from build123d import *

# Parameters (mm, degrees)
SKETCH2_W           = 208
SKETCH2_H           = 54
BOSS_EXTRUDE1_DEPTH = 10
SKETCH4_W           = 139
SKETCH4_H           = 54
CUT_EXTRUDE1_DEPTH  = 8
SKETCH3_W           = 40
SKETCH3_H           = 41
CUT_EXTRUDE2_DEPTH  = 8
SKETCH6_W           = 25
SKETCH6_H           = 54
BOSS_EXTRUDE2_DEPTH = 5
SKETCH7_W           = 20
SKETCH7_H           = 50
CUT_EXTRUDE3_DEPTH  = 1.5


with BuildPart() as part:
    # Sketch2 → Boss-Extrude1 (new body)
    with BuildSketch(Plane(origin=(0, 0, 0), x_dir=(1, 0, 0), z_dir=(0, 1, 0))):
        Rectangle(SKETCH2_W, SKETCH2_H)
    extrude(amount=BOSS_EXTRUDE1_DEPTH)

    # Sketch4 → Cut-Extrude1 (cut)
    with BuildSketch(Plane(origin=(0, 10, 0), x_dir=(1, 0, 0), z_dir=(0, 1, 0))):
        with Locations((-9.5, 0)):
            Rectangle(SKETCH4_W, SKETCH4_H)
    extrude(amount=-CUT_EXTRUDE1_DEPTH, mode=Mode.SUBTRACT)

    # Sketch3 → Cut-Extrude2 (cut)
    with BuildSketch(Plane(origin=(0, 10, 0), x_dir=(1, 0, 0), z_dir=(0, 1, 0))):
        with Locations((82, 2)):
            Rectangle(SKETCH3_W, SKETCH3_H)
    extrude(amount=-CUT_EXTRUDE2_DEPTH, mode=Mode.SUBTRACT)

    # Sketch6 → Boss-Extrude2 (add)
    with BuildSketch(Plane(origin=(0, 10, 0), x_dir=(1, 0, 0), z_dir=(0, 1, 0))):
        with Locations((-91.5, 0)):
            Rectangle(SKETCH6_W, SKETCH6_H)
    extrude(amount=BOSS_EXTRUDE2_DEPTH)

    # Sketch7 → Cut-Extrude3 (cut)
    with BuildSketch(Plane(origin=(0, 15, 0), x_dir=(1, 0, 0), z_dir=(0, 1, 0))):
        with Locations((-92, 0)):
            Rectangle(SKETCH7_W, SKETCH7_H)
    extrude(amount=-CUT_EXTRUDE3_DEPTH, mode=Mode.SUBTRACT)


solid = part.part
The listing builds one solid part. Answer for the finished solid, in the listing's coordinates (mm). A direction names the side the tool comes from. Give positions to 0.01 mm unless a question says otherwise; leave off trailing zeros. Loops run counter-clockwise (first coordinate to the right, second up) from the corner with the lowest first, then second, coordinate; pieces in that order, holes last.
Item 1: A tool of negligible diameter and unlimited length cuts with its end or side. For faces 1 (the flat face through (82, 10, 20)), 2 (the flat face through (82, 6, 18.5)), 3 (the flat face through (-79, 8, 0)), from which of +Z, -Z, +X, -X, +Y, -Y can it reach the whole face along a straight path? Write none if from no direction.
Derived:
face 1: +Z, -Z, +X, +Y
face 2: +Y
face 3: +Z, -Z, +Y
Item 2: Determine the mould class of faces 4 (the flat face through (82, 2, -2)), 5 (the flat face through (60, 6, 0)), 6 (the flat face through (0, 1, -27)) for opening direction Z: +Z half, -Z half, draft (parallel to the pull), parting line (faces both ways), or undercut.
Derived:
face 4: undercut
face 5: draft
face 6: -Z half
Item 3: Each of these flat-tipped pins is pushed along its axis until it touches: pin 1 Ø12 at (x, z) = (-83, -3) entering from +Y; pin 2 Ø10 at (x, z) = (-91, 6) entering from +Y; pin 3 Ø20 at (x, z) = (81.5, 5) entering from +Y; pin 4 Ø1.6 at (y, z) = (14, 3) entering from +X. Where does it stop, or does it pass through?
Derived:
pin 1: stops at y = 15
pin 2: stops at y = 13.5
pin 3: stops at y = 2
pin 4: stops at x = -79
Item 4: A cutting plane is placed at B-B (x = 86). Give the vertices of the cut face in (y, z), then the cut area to 3 significant figures.
Derived:
outline: (0, -27) - (10, -27) - (10, -22.5) - (2, -22.5) - (2, 18.5) - (10, 18.5) - (10, 27) - (0, 27) - close
area: 212 mm2
Item 5: A cutting plane is placed at D-D (z = -12). Give the vertices of the cut face in (x, y).
Derived:
outline: (-104, 0) - (104, 0) - (104, 10) - (102, 10) - (102, 2) - (62, 2) - (62, 10) - (60, 10) - (60, 2) - (-79, 2) - (-79, 15) - (-82, 15) - (-82, 13.5) - (-102, 13.5) - (-102, 15) - (-104, 15) - close
Item 6: A cutting plane is placed at A-A (y = 5.25). Give the vertices of the cut face in (x, z).
Derived:
outline: (-104, -27) - (-79, -27) - (-79, 27) - (-104, 27) - close; (60, -27) - (104, -27) - (104, 27) - (60, 27) - close; hole (62, -22.5) - (102, -22.5) - (102, 18.5) - (62, 18.5) - close
Item 7: Find the intervals of material crossed by line 1 along X through (y, z) = (9.25, -15.5); line 2 along X through (y, z) = (9.25, 25.5); line 3 along Z through (x, y) = (70, 6.75), in increasing order.
Derived:
line 1: x = -104 to -79, 60 to 62, 102 to 104
line 2: x = -104 to -79, 60 to 104
line 3: z = -27 to -22.5, 18.5 to 27
Item 8: A cutting plane is placed at C-C (z = 23). Give the vertices of the cut face in (x, y).
Derived:
outline: (-104, 0) - (104, 0) - (104, 10) - (60, 10) - (60, 2) - (-79, 2) - (-79, 15) - (-82, 15) - (-82, 13.5) - (-102, 13.5) - (-102, 15) - (-104, 15) - close
